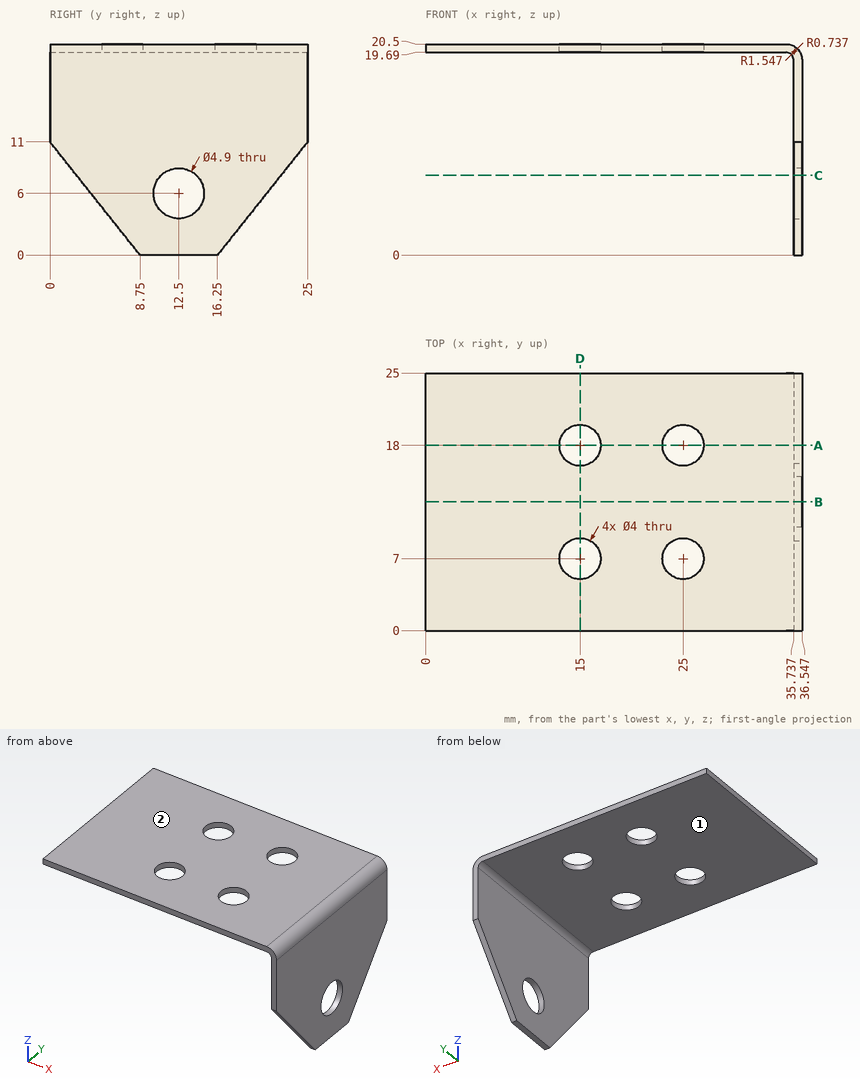
Design review of the part shown in the three views and the two pictorial views. Dimensions are in mm from the part's minimum x, y and z. A direction names the side the tool comes from. Coordinates: 2 decimals unless noted, no trailing zeros. Loops run counter-clockwise (first coordinate to the right, second up) from the corner with the lowest first, then second, coordinate; pieces in that order, holes last. Notation, with made-up numbers: M 20,49 L 62,49 A17 cw 62,68 Z; hole C 13.25,21.25 d9. An arc over 180 degrees is marked long. Put each result on its own line as item: value. Start each with the question number.
Q1. Wall thickness on line 1 (Y direction, x = 25, z = 20.1); line 2 (X direction, y = 20.25, z = 11.75); line 3 (Z direction, x = 5, y = 23.75): over which ranges is each line inside the solid? List them lowest first.
Q2. Clearance check with flat-ended pins moving along their axes: pin 1 (3.5 mm diameter, centred on x = 15, y = 18, fed in from -Z); pin 2 (2 mm diameter, centred on y = 15, z = 5, fed in from -X); pin 3 (1 mm diameter, centred on x = 19, y = 9.5, fed in from -Z). State where each tip first meets the part, or that it passes through.
Q3. Add section C-C (z = 7.75). Write out the cut boundary in (x, y) (1 decimal).
Q4. Add section A-A (y = 18). Write out the cut boundary in (x, z).
Q5. Add section D-D (x = 15). Write out the cut boundary in (y, z).
Q6. Add section B-B (y = 12.5). Write out the cut boundary in (x, z).
Q7. For the marked faces 1 and 2, list the 3-axis set-ups (+Z, -Z, +X, -X, +Y, -Y) from which the entire face can be reached by the end or side of a thin tool; tool diameter is ignored.
Answers:
1. line 1: y = 0 to 5, 9 to 16, 20 to 25
1. line 2: x = 35.74 to 36.55
1. line 3: z = 19.69 to 20.5
2. pin 1: passes through
2. pin 2: stops at x = 35.74
2. pin 3: stops at z = 19.69
3. outline: M 35.7,2.6 L 36.5,2.6 L 36.5,10.8 L 35.7,10.8 Z; M 35.7,14.2 L 36.5,14.2 L 36.5,22.4 L 35.7,22.4 Z
4. outline: M 0,19.69 L 13,19.69 L 13,20.5 L 0,20.5 Z; M 17,19.69 L 23,19.69 L 23,20.5 L 17,20.5 Z; M 27,19.69 L 35,19.69 A0.74 cw 35.74,18.95 L 35.74,2.2 L 36.55,2.2 L 36.55,18.95 A1.55 ccw 35,20.5 L 27,20.5 Z
5. outline: M 0,19.69 L 5,19.69 L 5,20.5 L 0,20.5 Z; M 9,19.69 L 16,19.69 L 16,20.5 L 9,20.5 Z; M 20,19.69 L 25,19.69 L 25,20.5 L 20,20.5 Z
6. outline: M 0,19.69 L 35,19.69 A0.74 cw 35.74,18.95 L 35.74,8.45 L 36.55,8.45 L 36.55,18.95 A1.55 ccw 35,20.5 L 0,20.5 Z; M 35.74,0 L 36.55,0 L 36.55,3.55 L 35.74,3.55 Z
7. face 1: -Z, -X, +Y, -Y
7. face 2: +Z, +X, -X, +Y, -Y
